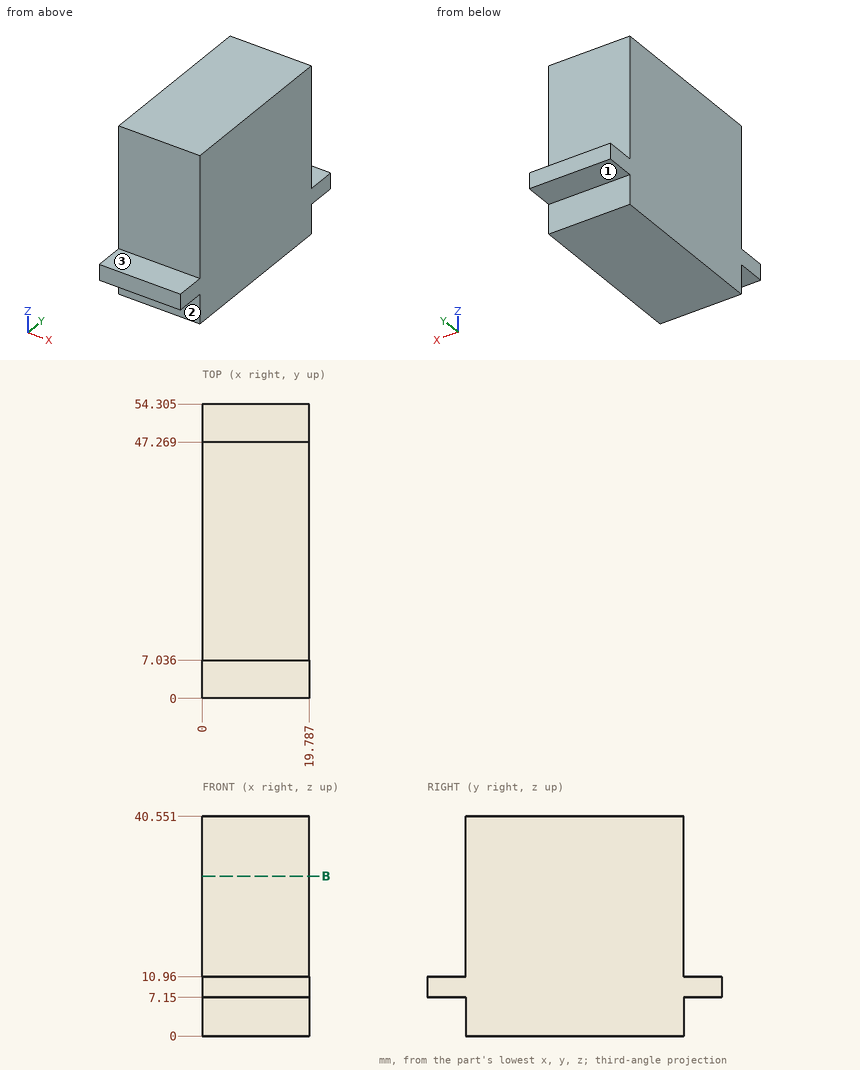
Design review of the part shown in the three views and the two pictorial views. Dimensions are in mm from the part's minimum x, y and z. A direction names the side the tool comes from. Round coordinates to 2 decimals unless told otherwise and drop trailing zeros. Write each loop counter-clockwise with the first axis right and the second up, starting at its lowest first coordinate (ties: lowest second). Pieces come first, ordered by that corner, then holes. Notation, with made-up numbers: (5, 7) - (29, 7) arc R27 cw to (29, 41) - close; hole circle Ø1 at (44, -33). An arc over 180 degrees is marked (long way). Return JSON: item names as keys, results as strings. Group by question number.
Item 1: Insertion check: P1, Ø2, axis at x = 4.5, z = 15, coming from the -Y side; P2, Ø6, axis at x = 10.5, y = 27, coming from the -Z side; P3, Ø8, axis at x = 13, z = 2, coming from the +Y side; P4, Ø2, axis at x = 9, y = 2, coming from the -Z side. Each pin has a flat end and moves straight along its axis. Give the tip position at first contact, or say it passes through.
Item 2: For probe 1 along Y at (x, z) = (6.5, 35) (1 decimal), list the stretches that pass through material, from the lowest coordinate up. Write a range as [from, to].
Item 3: We need section B-B on z = 29.5. Write out the cut boundary in (x, y) (1 decimal), and give its area (3 significant figures).
Item 4: Machinability: for the marked faces 1, 2 and 3, which of the approach directions +Z, -Z, +X, -X, +Y, -Y give a long, thin tool a straight path to every point of the face, cutting with its end or side? Answer none if there is none.
Model answer:
{
 "1": {"P1": "stops at y = 7.04", "P2": "stops at z = 0", "P3": "stops at y = 47.27", "P4": "stops at z = 7.15"},
 "2": {"probe 1": "y = [7, 47.3]"},
 "3": {"outline": "(0, 7) - (19.8, 7) - (19.8, 47.3) - (0, 47.3) - close", "area": "796 mm²"},
 "4": {"face 1": "-Z, +X, -X, +Y", "face 2": "-Z, +X, -X, -Y", "face 3": "+Z, +X, -X, -Y"}
}
